Part model, mm, in its own coordinate system. Give positions to 0.01 mm unless a question says otherwise; leave off trailing zeros. Loops run counter-clockwise (first coordinate to the right, second up) from the corner with the lowest first, then second, coordinate; pieces in that order, holes last. Notation, with made-up numbers: M -3.5,-9.5 L 1.5,-9.5 A16 ccw 1.5,-2.5 Z; hole C 39,86.25 d3. An arc over 180 degrees is marked long. Answer in a Markdown table with one row per item.
from build123d import *

# Parameters (mm, degrees)
ESQUISSE1_R             = 5
BOSS_EXTRU_1_DEPTH      = 820
ESQUISSE2_R             = 10
BOSS_EXTRU_2_DEPTH      = 500
CHANFREIN1_SIZE         = 10
CHANFREIN1_SIZE_2       = 43.314758743
ESQUISSE3_R             = 4
ENL_V_MAT_EXTRU_1_DEPTH = 821.121942153


with BuildPart() as part:
    # Esquisse1 → Boss.-Extru.1 (new body)
    with BuildSketch(Plane(origin=(0, 0, 0), x_dir=(1, 0, 0), z_dir=(0, 1, 0))):
        with Locations(Location((0, 0, 0), (0, 0, 270))):
            Circle(ESQUISSE1_R)
    extrude(amount=BOSS_EXTRU_1_DEPTH)

    # Esquisse2 → Boss.-Extru.2 (add)
    with BuildSketch(Plane(origin=(0, 0, 0), x_dir=(1, 0, 0), z_dir=(0, 1, 0))):
        with Locations(Location((0, 0, 0), (0, 0, 270))):
            Circle(ESQUISSE2_R)
    extrude(amount=BOSS_EXTRU_2_DEPTH)

    # Chanfrein1
    # the kernel refuses this chamfer: 43.314758743, 10 mm, written as the material it adds along each edge
    with BuildSketch(Plane(origin=(0, 500, 0), x_dir=(0, 0, 1), z_dir=(1, 0, 0))) as chanfrein1_piece_1_section:
        Polygon((5 + CHANFREIN1_SIZE, 0), (5, -CHANFREIN1_SIZE_2), (5, 0), align=None)
    chanfrein1_piece_1 = revolve(axis=Axis((0, 500, 0), (0, -1, 0)), mode=Mode.PRIVATE)
    chanfrein1_piece_1 = chanfrein1_piece_1 & Plane(origin=(0, 533.283833366, 0), x_dir=(0, 0, 1), z_dir=(0, -1, 0)) * Cylinder(10, 174, mode=Mode.PRIVATE)
    add(chanfrein1_piece_1)

    # Esquisse3 → Enlèv. mat.-Extru.1 (cut, through all)
    with BuildSketch(Plane(origin=(0, 820, 0), x_dir=(1, 0, 0), z_dir=(0, 1, 0))):
        with Locations(Location((0, 0, 0), (0, 0, 270))):
            Circle(ESQUISSE3_R)
    extrude(amount=-ENL_V_MAT_EXTRU_1_DEPTH, mode=Mode.SUBTRACT)


solid = part.part
(1) Saw through at A-A (z = 0). Write the cut outline in (x, y), plus the area to 3 significant figures.
Recorded:
| item | result |
|---|---|
| outline | M -10,0 L -4,0 L -4,820 L -5,820 L -5,543.31 L -10,521.66 Z; M 4,0 L 10,0 L 10,521.66 L 5,543.31 L 5,820 L 4,820 Z |
| area | 6,960 mm^2 |
(2) Pin check, flat tips, straight feed: pin 1 Ø1.5 at (y, z) = (116, -5) entering from +X; pin 2 Ø2 at (y, z) = (673.5, 2) entering from +X; pin 3 Ø7 at (x, z) = (0, 0) entering from -Y; pin 4 Ø2 at (x, y) = (5, 240) entering from -Z. Stop position of each tip, or through.
Recorded:
| item | result |
|---|---|
| pin 1 | stops at x = 9.05 |
| pin 2 | stops at x = 4.9 |
| pin 3 | passes through |
| pin 4 | stops at z = -9.17 |
(3) Saw through at D-D (y = 655.5). Write the cut outline in (x, z).
Recorded:
| item | result |
|---|---|
| outline | C 0,0 d10; hole C 0,0 d8 |
(4) Drill centre lines: line 1 along X through (y, z) = (503.5, 0); line 2 along X through (y, z) = (612.5, 0); line 3 along Z through (x, y) = (1, 467.5). Where is each one in solid material? Low to high.
Recorded:
| item | result |
|---|---|
| line 1 | x = -10 to -4, 4 to 10 |
| line 2 | x = -5 to -4, 4 to 5 |
| line 3 | z = -9.95 to -3.87, 3.87 to 9.95 |
(5) Saw through at B-B (x = 0). Write the cut outline in (y, z).
Recorded:
| item | result |
|---|---|
| outline | M 0,-10 L 521.66,-10 L 543.31,-5 L 820,-5 L 820,-4 L 0,-4 Z; M 0,4 L 820,4 L 820,5 L 543.31,5 L 521.66,10 L 0,10 Z |
(6) Saw through at C-C (y = 321.5). Write the cut outline in (x, z), plus the area to 3 significant figures.
Recorded:
| item | result |
|---|---|
| outline | C 0,0 d20; hole C 0,0 d8 |
| area | 264 mm^2 |
